The listing builds one solid part. Answer for the finished solid, in the listing's coordinates (mm). A direction names the side the tool comes from. Coordinates: 2 decimals unless noted, no trailing zeros. Order: outer loops, then holes, each group sorted by start corner. A loop starts at its lowest first (then second) coordinate and runs counter-clockwise, first axis right, second up. Notation, with made-up numbers: (32, 60.5) -> (60, 60.5) arc R11 cw to (60, 64.5) -> close; hole circle Ø1 at (74, 31.5). An arc over 180 degrees is marked (long way). Write item = value, one per line. Start each with the question number.
```python
from build123d import *

# Parameters (mm, degrees)
EXTRUDE_1_DEPTH = 2
SKETCH_2_R      = 3.5
SKETCH_2_R_2    = 2.5
EXTRUDE_2_DEPTH = 3


with BuildPart() as part:
    # 草图1 → 凸台-拉伸1 (new body)
    with BuildSketch(Plane.XY):
        with BuildLine():
            Line((-4.96903995, 0.555555556), (-2.484519975, 22.777777778))
            ThreePointArc((-2.484519975, 22.777777778), (0, 25), (2.484519975, 22.777777778))
            Line((2.484519975, 22.777777778), (4.96903995, 0.555555556))
            ThreePointArc((4.96903995, 0.555555556), (0, -5), (-4.96903995, 0.555555556))
        make_face()
    extrude(amount=EXTRUDE_1_DEPTH)

    # 草图2 → 凸台-拉伸2 (add)
    with BuildSketch(Plane.XY.offset(2)):
        Circle(SKETCH_2_R)
        Circle(SKETCH_2_R_2, mode=Mode.SUBTRACT)
    extrude(amount=EXTRUDE_2_DEPTH)


solid = part.part
```
Item 1: Section A-A, the plane y = 0 is taken. Give the vertices of the cut face in (x, z), then the cut area to 3 significant figures.
Item 2: Which of the six approach directions +Z, -Z, +X, -X, +Y, -Y give full straight-line access (tool end or side, diameter ignored) to faces 1 (the flat face through (-3.744, 11.511, 0.986)), 2 (the cylindrical face through (3.233, -1.341, 3.479))?
Item 3: Consider probe 1 along Y at (x, z) = (0, 3.45); probe 2 along Z at (x, y) = (-2.75, 15); probe 3 along Y at (x, z) = (-1.5, 3.4). Determine where each line is inside the solid, lowest interval first.
Item 4: Section B-B, the plane x = 0 is taken. Give the vertices of the cut face in (y, z), then the cut area to 3 significant figures.
Item 5: Section D-D, the plane z = 0.8 is taken. Give the vertices of the cut face in (x, y), then the cut area to 3 significant figures.
Item 6: Each of these flat-tipped pins is pushed along its axis until it touches: pin 1 (1.5 mm diameter, centred on x = -0.5, y = -1, fed in from +Z); pin 2 (5 mm diameter, centred on x = 3.5, y = 12.5, fed in from -Z); pin 3 (2 mm diameter, centred on y = 13.5, z = 1.5, fed in from -X); pin 4 (2 mm diameter, centred on x = 2.5, z = 3.5, fed in from -Y). Where does it stop, or does it pass through?
Item 7: Section C-C, the plane z = 4.6 is taken. Give the vertices of the cut face in (x, y), then the cut area to 3 significant figures.
Item 8: For a pull along X with two mould halves and no side action, classify faces 3 (the cylindrical face through (0, 25, 1)), 4 (the flat face through (0, 7, 0)), 5 (the flat face through (0, 0, 2)), 6 (the flat face through (3.71, 11.82, 0.99)) as pulls with the +X half, pulls with the -X half, needs draft (parallel to the pull), parting line crosses it, or undercut.
A:
q1.outline = (-5, 0) -> (5, 0) -> (5, 2) -> (3.5, 2) -> (3.5, 5) -> (2.5, 5) -> (2.5, 2) -> (-2.5, 2) -> (-2.5, 5) -> (-3.5, 5) -> (-3.5, 2) -> (-5, 2) -> close
q1.area = 26.0 mm^2
q2.face_1 = +Z, -Z, -X, +Y
q2.face_2 = +Z
q3.probe_1 = -3.5 to -2.5, 2.5 to 3.5
q3.probe_2 = 0 to 2
q3.probe_3 = -3.16 to -2, 2 to 3.16
q4.outline = (-5, 0) -> (25, 0) -> (25, 2) -> (3.5, 2) -> (3.5, 5) -> (2.5, 5) -> (2.5, 2) -> (-2.5, 2) -> (-2.5, 5) -> (-3.5, 5) -> (-3.5, 2) -> (-5, 2) -> close
q4.area = 66.0 mm^2
q5.outline = (-4.97, 0.56) arc R5 ccw (long way) to (4.97, 0.56) -> (2.48, 22.78) arc R2.5 ccw to (-2.48, 22.78) -> close
q5.area = 219 mm^2
q6.pin_1 = 2
q6.pin_2 = 0
q6.pin_3 = -3.63
q6.pin_4 = -3.16
q7.outline = circle Ø7 at (0, 0); hole circle Ø5 at (0, 0)
q7.area = 18.8 mm^2
q8.face_3 = parting line crosses it
q8.face_4 = needs draft
q8.face_5 = undercut
q8.face_6 = pulls with the +X half
